```python
from build123d import *

# Parameters (mm, degrees)
SKETCH1_R           = 1.5
BOSS_EXTRUDE1_DEPTH = 5
FILLET1_R           = 3
CUT_EXTRUDE2_REACH  = 7
SKETCH7_R           = 1.5


with BuildPart() as part:
    # Sketch1 → Boss-Extrude1 (new body)
    with BuildSketch(Plane(origin=(0, 0, 0), x_dir=(0, 0, -1), z_dir=(1, 0, 0))):
        with BuildLine():
            Line((0, 0), (0, 15))
            Line((0, 15), (4.951340344, 15.695865505))
            ThreePointArc((4.951340344, 15.695865505), (27.926864621, 22.182944056), (48.325875811, 34.586058439))
            ThreePointArc((48.325875811, 34.586058439), (59.519665724, 53.069681974), (56.412643103, 74.454061366))
            Line((56.412643103, 74.454061366), (43.267439345, 99.176593966))
            Line((43.267439345, 99.176593966), (65.341129166, 110.913383036))
            Line((65.341129166, 110.913383036), (90.292806812, 85.883380245))
            ThreePointArc((90.292806812, 85.883380245), (91.119279883, 84.674725039), (91.455424552, 83.249624372))
            Line((91.455424552, 83.249624372), (94.07546653, 28.221444591))
            Line((94.07546653, 28.221444591), (94.36203286, 22.202753427))
            Line((94.36203286, 22.202753427), (22, 12.032932928))
            Line((22, 12.032932928), (22, 0))
            Line((22, 0), (0, 0))
        make_face()
        with Locations((4, 3)):
            Circle(SKETCH1_R, mode=Mode.SUBTRACT)
        with Locations((18, 3)):
            Circle(SKETCH1_R, mode=Mode.SUBTRACT)
        with Locations((67, 105)):
            Circle(SKETCH1_R, mode=Mode.SUBTRACT)
        with BuildLine():
            Line((37.734060935, 20.303176421), (88.108596969, 27.382855762))
            Line((88.108596969, 27.382855762), (85.763043155, 76.646019476))
            ThreePointArc((85.763043155, 76.646019476), (80.419740702, 73.76043279), (74.648335848, 71.871417797))
            Line((74.648335848, 71.871417797), (64.774649495, 69.591897689))
            ThreePointArc((64.774649495, 69.591897689), (64.35710923, 47.870362906), (52.107292501, 29.927637267))
            ThreePointArc((52.107292501, 29.927637267), (45.141760841, 24.785238396), (37.734060935, 20.303176421))
        make_face(mode=Mode.SUBTRACT)
        with BuildLine():
            Line((83.108700039, 84.591428686), (64.231449963, 103.527935833))
            Line((64.231449963, 103.527935833), (51.381954278, 96.695737786))
            Line((51.381954278, 96.695737786), (61.793684809, 77.114120627))
            Line((61.793684809, 77.114120627), (72.848727413, 79.666378316))
            ThreePointArc((72.848727413, 79.666378316), (78.251497028, 81.560635362), (83.108700039, 84.591428686))
        make_face(mode=Mode.SUBTRACT)
        with BuildLine():
            ThreePointArc((74.085958212, 74.307342959), (81.788354228, 77.187150825), (88.482948342, 81.962358399))
            ThreePointArc((88.482948342, 81.962358399), (88.556981354, 84.082386492), (86.436953262, 84.156419504))
            ThreePointArc((86.436953262, 84.156419504), (80.379939539, 79.835993604), (73.411105049, 77.230453154))
            ThreePointArc((73.411105049, 77.230453154), (72.286976533, 75.431471475), (74.085958212, 74.307342959))
        make_face(mode=Mode.SUBTRACT)
    extrude(amount=BOSS_EXTRUDE1_DEPTH)

    # Fillet1
    fillet1_edges = [part.edges().sort_by_distance(p)[0] for p in [
        (2.5, 15, 0),
        (2.5, 99.176593966, -43.267439345),
        (2.5, 110.913383036, -65.341129166),
        (2.5, 22.202753427, -94.36203286),
        (2.5, 12.032932928, -22),
        (2.5, 20.303176421, -37.734060935),
        (2.5, 27.382855762, -88.108596969),
        (2.5, 76.646019476, -85.763043155),
        (2.5, 69.591897689, -64.774649495),
        (2.5, 84.591428686, -83.108700039),
        (2.5, 103.527935833, -64.231449963),
        (2.5, 96.695737786, -51.381954278),
        (2.5, 77.114120627, -61.793684809),
    ]]
    fillet(fillet1_edges, radius=FILLET1_R)

    # Sketch7 → Cut-Extrude2 (cut, up to next)
    with BuildSketch(Plane(origin=(5, 0, 0), x_dir=(0, 0, -1), z_dir=(1, 0, 0)), mode=Mode.PRIVATE) as cut_extrude2_sk1:
        with Locations((31.81923079, 16.442418537)):
            Circle(SKETCH7_R)
    cut_extrude2_tool1 = extrude(cut_extrude2_sk1.sketch, amount=-CUT_EXTRUDE2_REACH, mode=Mode.PRIVATE) & part.part
    add(cut_extrude2_tool1.solids().sort_by_distance((5, 16.442419, -31.819231))[0], mode=Mode.SUBTRACT)
    # Sketch7 → Cut-Extrude2 (cut, up to next)
    with BuildSketch(Plane(origin=(5, 0, 0), x_dir=(0, 0, -1), z_dir=(1, 0, 0)), mode=Mode.PRIVATE) as cut_extrude2_sk2:
        with Locations((91.235314915, 24.792804595)):
            Circle(SKETCH7_R)
    cut_extrude2_tool2 = extrude(cut_extrude2_sk2.sketch, amount=-CUT_EXTRUDE2_REACH, mode=Mode.PRIVATE) & part.part
    add(cut_extrude2_tool2.solids().sort_by_distance((5, 24.792805, -91.235315))[0], mode=Mode.SUBTRACT)


solid = part.part
```
Work out the finished part from the listing and answer in its coordinate system (mm). A direction names the side the tool comes from. Round coordinates to 2 decimals unless told otherwise and drop trailing zeros. Write each loop counter-clockwise with the first axis right and the second up, starting at its lowest first coordinate (ties: lowest second). Pieces come first, ordered by that corner, then holes. Notation, with made-up numbers: (-28, 49) -> (-3, 49) arc R17 cw to (-3, 72) -> close; hole circle Ø5 at (53, 21). An arc over 180 degrees is marked (long way). Write each question's results on one line, items separated by ' | '.
Q1. Which of the six approach directions +Z, -Z, +X, -X, +Y, -Y give full straight-line access (tool end or side, diameter ignored) to faces 1 (the flat face through (2, 5, -22)), 2 (the cylindrical face through (2.535, 102.798, -64.149)), 3 (the flat face through (2, 6, 0))?
Data:
face 1: -Z, +X, -X, -Y | face 2: +X, -X | face 3: +Z, +X, -X, +Y, -Y
Q2. Flat-ended cylindrical pins translate along their axes: P1, Ø2.5, axis at y = 3, z = -4, coming from the +X side; P2, Ø3, axis at x = 1, y = 60, coming from the -Z side. Find the tip coordinate at first contact, or state that the pin passes through.
Data:
P1: through | P2: z = -92.63
Q3. Determine the mould class of faces 4 (the flat face through (2, 0, -11)), 5 (the cylindrical face through (2.46, 84.06, -88.58)), 6 (the cylindrical face through (2.465, 84.694, -91.111)) for opening direction Z: released by +Z, released by -Z, zero draft, split by the parting line, or undercut.
Data:
face 4: zero draft | face 5: undercut | face 6: released by -Z
Q4. Section B-B, the plane y = 44.5 is taken. Write down the section's boundary in (x, z), then the cut area to 3 significant figures.
Data:
outline: (0, -93.3) -> (5, -93.3) -> (5, -87.29) -> (0, -87.29) -> close; (0, -63.1) -> (5, -63.1) -> (5, -56.46) -> (0, -56.46) -> close | area: 63.2 mm^2
Q5. Section C-C, the plane x = 2.6 is taken. Give the number of separate pieces and of enclosed holes in the cut face, then the cut area to 3 significant figures.
Data:
separate pieces: 1 | enclosed holes: 8 | area: 2,190 mm^2
Q6. Section A-A, the plane y = 3 is taken. Write down the section's boundary in (x, z).
Data:
outline: (0, -22) -> (5, -22) -> (5, -19.5) -> (0, -19.5) -> close; (0, -16.5) -> (5, -16.5) -> (5, -5.5) -> (0, -5.5) -> close; (0, -2.5) -> (5, -2.5) -> (5, 0) -> (0, 0) -> close
Q7. Straight lines are drawn through the part: line 1 along Y through (x, z) = (3.55, -53); line 2 along Z through (x, y) = (0.9, 82.5); line 3 along Y through (x, z) = (3.5, -57). For each, find the intervals that lie inside material, in ascending order. Write a range as [from, to].
Data:
line 1: [16.39, 22.45], [30.68, 39.26], [80.87, 93.65], [97.2, 104.35] | line 2: [-91.49, -88.85], [-84.49, -80.02], [-58.93, -52.13] | line 3: [16.95, 23.01], [34.69, 45.57], [73.29, 86.13], [99.68, 106.48]
